For this review, use the dimensioned drawing (mm, ordinates from the lowest corner) and the shaded views. Coordinates: 2 decimals unless noted, no trailing zeros. Order: outer loops, then holes, each group sorted by start corner. A loop starts at its lowest first (then second) coordinate and runs counter-clockwise, first axis right, second up. Notation, with made-up numbers: M -8.5,21.25 L 1.5,21.25 A23 ccw 1.5,53.25 Z; hole C 15.25,71.5 d7. An arc over 180 degrees is marked long. Answer in a Markdown table with one row per item.
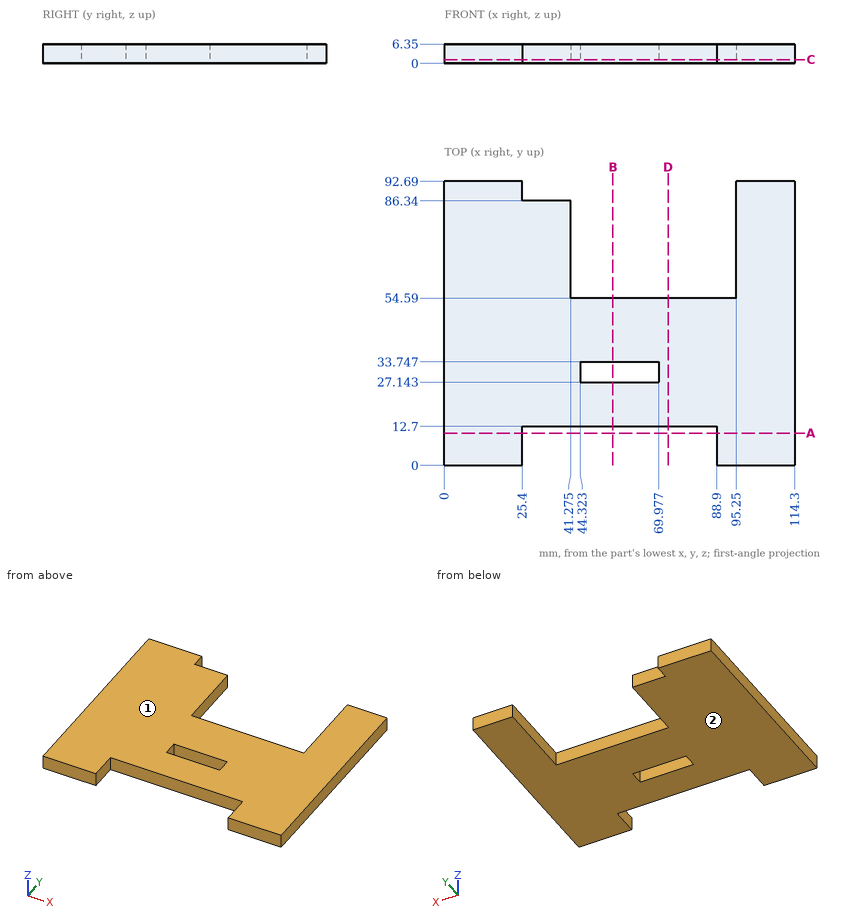
(1) To check wall thickness, follow line 1 (X direction, y = 11, z = 5.5); line 2 (X direction, y = 55, z = 5.25) (3 decimals); line 3 (Y direction, x = 44.5, z = 3.75). State the ranges of each line that lie inside material, in increasing order. Write a range as [from, to].
Report:
| item | result |
|---|---|
| line 1 | [0, 25.4], [88.9, 114.3] |
| line 2 | [0, 41.275], [95.25, 114.3] |
| line 3 | [12.7, 27.14], [33.75, 54.59] |
(2) The part is to be moulded in two halves that separate along Z. For the marked faces 1 and 2, say which applies: +Z half, -Z half, draft (parallel to the pull), parting line (faces both ways), or undercut.
Report:
| item | result |
|---|---|
| face 1 | +Z half |
| face 2 | -Z half |
(3) Take a section at D-D (x = 73). Write out the cut boundary in (y, z).
Report:
| item | result |
|---|---|
| outline | M 12.7,0 L 54.59,0 L 54.59,6.35 L 12.7,6.35 Z |
(4) Take a section at A-A (y = 10.5). Write out the cut boundary in (x, z).
Report:
| item | result |
|---|---|
| outline | M 0,0 L 25.4,0 L 25.4,6.35 L 0,6.35 Z; M 88.9,0 L 114.3,0 L 114.3,6.35 L 88.9,6.35 Z |
(5) Take a section at C-C (z = 1.25). Write out the cut boundary in (x, y) (3 decimals), then the cut area to 3 significant figures.
Report:
| item | result |
|---|---|
| outline | M 0,0 L 25.4,0 L 25.4,12.7 L 88.9,12.7 L 88.9,0 L 114.3,0 L 114.3,92.69 L 95.25,92.69 L 95.25,54.59 L 41.275,54.59 L 41.275,86.34 L 25.4,86.34 L 25.4,92.69 L 0,92.69 Z; hole M 44.323,27.143 L 69.977,27.143 L 69.977,33.747 L 44.323,33.747 Z |
| area | 7,460 mm^2 |
(6) Insertion check: P1, Ø3, axis at x = 31, z = 1.5, coming from the +Y side; P2, Ø1.9, axis at x = 53.5, z = 2.5, coming from the -Y side; P3, Ø3, axis at x = 65.5, z = 2, coming from the +Y side. Each pin has a flat end and moves straight along its axis. Give the tip position at first contact, or say it passes through.
Report:
| item | result |
|---|---|
| P1 | y = 86.34 |
| P2 | y = 12.7 |
| P3 | y = 54.59 |
(7) Take a section at B-B (x = 55). Write out the cut boundary in (y, z), then the cut area to 3 significant figures.
Report:
| item | result |
|---|---|
| outline | M 12.7,0 L 27.14,0 L 27.14,6.35 L 12.7,6.35 Z; M 33.75,0 L 54.59,0 L 54.59,6.35 L 33.75,6.35 Z |
| area | 224 mm^2 |
